from build123d import *

# Parameters (mm, degrees)
F1_DEPTH = 63.5
F0_W     = 27.5913768614
F0_H     = 19.05
F2_DEPTH = 25.4
F3_DEPTH = 6.35


with BuildPart() as f1:
    # F0 (on Front) → F1 (new body, symmetric)
    with BuildSketch(Plane.XZ):
        Polygon((22.225, 9.525), (-41.275, 9.525), (-41.275, -9.525), (41.275, -9.525), (41.275, 9.525), align=None)
    extrude(amount=F1_DEPTH, both=True)

    # F0 (on Front) → F2 (join, symmetric)
    with BuildSketch(Plane.XZ):
        with BuildLine():
            Line((22.225, 46.0502), (22.225, 9.525))
            Line((22.225, 9.525), (41.275, 9.525))
            Line((41.275, 9.525), (41.275, 46.0502))
            ThreePointArc((41.275, 46.0502), (45.9246798487, 57.2755201513), (57.15, 61.9252))
            Line((57.15, 61.9252), (60.325, 61.9252))
            Line((60.325, 61.9252), (60.325, 80.9752))
            Line((60.325, 80.9752), (57.15, 80.9752))
            add(Edge.make_bspline(
                [(56.2404700013, 80.96335483), (56.5431683561, 80.9684989137), (56.846346144, 80.9724501926), (57.15, 80.9752)],
                knots=[120.9786542661, 120.9786542661, 120.9786542661, 120.9786542661, 121.6248811101, 121.6248811101, 121.6248811101, 121.6248811101], degree=3))
            ThreePointArc((56.2404700013, 80.96335483), (32.1347950218, 70.4222156101), (22.225, 46.0502))
        make_face()
        with Locations((74.1206884307, 71.4502)):
            Rectangle(F0_W, F0_H)
        Polygon((60.325, 84.455), (60.325, 80.9752), (87.9163768614, 80.9752), (87.9163768614, 61.9252), (60.325, 61.9252), (60.325, 55.88), (111.125, 55.88), (111.125, 84.455), align=None)
    extrude(amount=F2_DEPTH, both=True)

    # F0 (on Front) → F3 (join, symmetric)
    with BuildSketch(Plane.XZ):
        with BuildLine():
            add(Edge.make_bspline(
                [(-41.275, 9.525), (-40.2919004024, 37.2334202637), (-0.4269989303, 80.0003426359), (56.2404700013, 80.96335483)],
                knots=[0, 0, 0, 0, 120.9786542661, 120.9786542661, 120.9786542661, 120.9786542661], degree=3))
            Line((-41.275, 9.525), (22.225, 9.525))
            Line((22.225, 9.525), (22.225, 46.0502))
            ThreePointArc((22.225, 46.0502), (32.1347950218, 70.4222156101), (56.2404700013, 80.96335483))
        make_face()
    extrude(amount=F3_DEPTH, both=True)


solid = f1.part
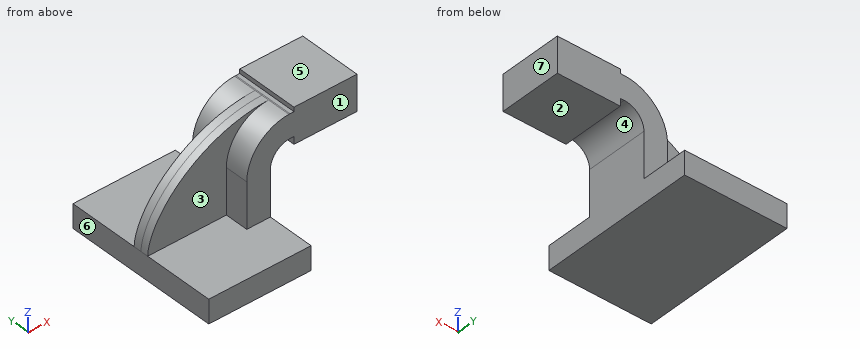
Check sheet for the modelled part. Datum: model origin and axes. Units: mm. Face numbers are marked on the shaded views. A direction names the side the tool comes from. Round coordinates to 2 decimals unless told otherwise and drop trailing zeros. Loops run counter-clockwise (first coordinate to the right, second up) from the corner with the lowest first, then second, coordinate; pieces in that order, holes last.
1. Set-up check for the marked faces 1, 2 and 3: record each of +Z, -Z, +X, -X, +Y, -Y from which the full face is reachable in a straight line by a thin tool's end or side.
2. Scan lines: probe 1 along X at (y, z) = (-49, -4) (3 decimals); probe 2 along Y at (x, z) = (96.5, 77.5); probe 3 along Z at (x, y) = (-24, -53) (3 decimals). Record each from-to range of solid material in increasing order.
3. Sectioned sample at B-B on y = -36.5. Record the boundary of the cut face in (x, z) (3 decimals), and give its area (3 significant figures).
4. Gauge pin test, flat ends, axial feed: pin 1 Ø1.5 at (y, z) = (10.5, 53.5) entering from -X; pin 2 Ø15 at (y, z) = (-16, 20) entering from -X (3 decimals); pin 3 Ø1 at (x, y) = (58.5, 7) entering from -Z. Record the tip position at first contact, or that the pin passes through.
5. Sectioned sample at A-A on z = 0. Record the boundary of the cut face in (x, y) (3 decimals), and give its area (3 significant figures).
6. Mould release check, pull along X, two halves, no side actions. Record for the marked faces 4, 5, 6 and 7: released by +X, released by -X, zero draft, split by the parting line, or undercut.
Recorded:
1. face 1: +Z, +X, -X, -Y
1. face 2: -Z, +X, +Y, -Y
1. face 3: +Z, -X, -Y
2. probe 1: x = -41.275 to 41.275
2. probe 2: y = -25.4 to 25.4
2. probe 3: z = -9.525 to 9.525
3. outline: (-41.275, -9.525) - (41.275, -9.525) - (41.275, 9.525) - (-41.275, 9.525) - close
3. area: 1,570 mm2
4. pin 1: stops at x = 22.87
4. pin 2: stops at x = 22.225
4. pin 3: stops at z = 61.93
5. outline: (-41.275, -63.5) - (41.275, -63.5) - (41.275, 63.5) - (-41.275, 63.5) - close
5. area: 10,500 mm2
6. face 4: undercut
6. face 5: zero draft
6. face 6: released by -X
6. face 7: released by +X
